Design review of the part built by this model. Coordinates are the model's own, in mm. A direction names the side the tool comes from. Give positions to 0.01 mm unless a question says otherwise; leave off trailing zeros. Write each loop counter-clockwise with the first axis right and the second up, starting at its lowest first coordinate (ties: lowest second). Pieces come first, ordered by that corner, then holes. Notation, with made-up numbers: (80, 19.5) - (95, 19.5) arc R20 ccw to (95, 45.5) - close; hole circle Ø2 at (-13.75, 17.25). An arc over 180 degrees is marked (long way). Use a Markdown table: item, result. Add a question column.
```python
from build123d import *

# Parameters (mm, degrees)
SKETCH1_R                   = 2.5
SKETCH1_R_2                 = 1.1
SHOULDER_SPACER_L9_DEPTH    = 9
LOWER_TORQUE_PILOT_D3_START = -1
SKETCH2_R                   = 1.5
SKETCH2_R_2                 = 1.1
LOWER_TORQUE_PILOT_D3_DEPTH = 1
UPPER_TORQUE_PILOT_D3_START = 9
SKETCH3_R                   = 1.5
SKETCH3_R_2                 = 1.1
UPPER_TORQUE_PILOT_D3_DEPTH = 1


with BuildPart() as part:
    # Sketch1 → Shoulder_Spacer_L9 (new body)
    with BuildSketch(Plane.XY):
        Circle(SKETCH1_R)
        Circle(SKETCH1_R_2, mode=Mode.SUBTRACT)
    extrude(amount=SHOULDER_SPACER_L9_DEPTH)

    # Sketch2 → Lower_Torque_Pilot_D3 (add)
    with BuildSketch(Plane.XY.offset(LOWER_TORQUE_PILOT_D3_START)):
        Circle(SKETCH2_R)
        Circle(SKETCH2_R_2, mode=Mode.SUBTRACT)
    extrude(amount=LOWER_TORQUE_PILOT_D3_DEPTH)

    # Sketch3 → Upper_Torque_Pilot_D3 (add)
    with BuildSketch(Plane.XY.offset(UPPER_TORQUE_PILOT_D3_START)):
        Circle(SKETCH3_R)
        Circle(SKETCH3_R_2, mode=Mode.SUBTRACT)
    extrude(amount=UPPER_TORQUE_PILOT_D3_DEPTH)


solid = part.part
```
(1) Mouldability with a two-part tool opening along X and no side actions: class faces 1 (the face through (-1.5, 0.07, 9.49)), 2 (the face through (0, -2, 0)), 3 (the face through (1.05, 0.33, 4.42)) as +X half, -X half, draft (parallel to the pull), parting line (faces both ways), or undercut.
(2) Insertion check: pin 1 (1.5 mm diameter, centred on x = -1.5, z = 0.5, fed in from +Y); pin 2 (1.5 mm diameter, centred on x = -1.5, z = 8, fed in from -Y); pin 3 (2 mm diameter, centred on y = -1, z = 2.5, fed in from -X). Each pin has a flat end and moves straight along its axis. Give the tip position at first contact, or say it passes through.
(3) Add section C-C (z = 8). State the section outline as (x, y) points, and give its area (3 significant figures).
(4) Tool access review of faces 4 (the face through (0, -2, 9)), 5 (the face through (-1.5, 0.07, -0.51)), 6 (the face through (-0.54, -2.44, 4.44)): name each direction out of +Z, -Z, +X, -X, +Y, -Y from which nothing blocks a thin tool from reaching the whole face with its end or side.
(5) For line 1 along Y through (x, z) = (0, 2); line 2 along Z through (x, y) = (-1.15, 1.3); line 3 along X through (y, z) = (-0.3, 8.25), list the stretches that pass through material, from the lowest coordinate up.
(6) Add section D-D (x = -1.25). State the section outline as (y, z) points.
(7) Add section A-A (x = 0). State the section outline as (y, z) points, and give its area (3 significant figures).
Answers follow:
| question | item | result |
|---|---|---|
| 1 | face 1 | parting line |
| 1 | face 2 | draft |
| 1 | face 3 | undercut |
| 2 | pin 1 | y = 2.38 |
| 2 | pin 2 | y = -2.38 |
| 2 | pin 3 | x = -2.5 |
| 3 | outline | circle Ø5 at (0, 0); hole circle Ø2.2 at (0, 0) |
| 3 | area | 15.8 mm^2 |
| 4 | face 4 | +Z |
| 4 | face 5 | -Z |
| 4 | face 6 | +Z, -Z |
| 5 | line 1 | -2.5 to -1.1, 1.1 to 2.5 |
| 5 | line 2 | 0 to 9 |
| 5 | line 3 | -2.48 to -1.06, 1.06 to 2.48 |
| 6 | outline | (-2.17, 0) - (-0.83, 0) - (-0.83, -1) - (0.83, -1) - (0.83, 0) - (2.17, 0) - (2.17, 9) - (0.83, 9) - (0.83, 10) - (-0.83, 10) - (-0.83, 9) - (-2.17, 9) - close |
| 7 | outline | (-2.5, 0) - (-1.5, 0) - (-1.5, -1) - (-1.1, -1) - (-1.1, 10) - (-1.5, 10) - (-1.5, 9) - (-2.5, 9) - close; (1.1, -1) - (1.5, -1) - (1.5, 0) - (2.5, 0) - (2.5, 9) - (1.5, 9) - (1.5, 10) - (1.1, 10) - close |
| 7 | area | 26.8 mm^2 |
